Read the model definition and answer for the solid it produces. Units are mm, in the model's axes. A direction names the side the tool comes from. Round coordinates to 2 decimals unless told otherwise and drop trailing zeros. Order: outer loops, then holes, each group sorted by start corner. A loop starts at its lowest first (then second) coordinate and runs counter-clockwise, first axis right, second up.
Autodesk Inventor part; units mm, degrees
ref_plane "YZ Plane" through (0, 0, 0) normal (1, 0, 0) x (0, 1, 0)
ref_plane "XZ Plane" through (0, 0, 0) normal (0, 1, 0) x (-1, 0, 0)
ref_plane "XY Plane" through (0, 0, 0) normal (0, 0, 1) x (1, 0, 0)
sketch "Sketch1" plane through (0, 0, 0) normal (0, 1, 0) x (-1, 0, 0)
  line L0 (-166.6875, 104.5) -> (166.6875, 104.5)
  line L1 (166.6875, -104.5) -> (-166.6875, -104.5)
  line L2 (-166.6875, 104.5) -> (166.6875, -104.5) construction
  line L3 (166.6875, 104.5) -> (-166.6875, -104.5) construction
  line L4 (166.6875, 88.5) -> (-166.6875, 88.5)
  line L5 (166.6875, -88.5) -> (-166.6875, -88.5)
  line L6 (120.9675, 104.5) -> (120.9675, -104.5)
  line L7 (-120.9675, 104.5) -> (-120.9675, -104.5)
  line L8 (-109.9675, 104.5) -> (-109.9675, -104.5)
  line L9 (-131.9675, 104.5) -> (-131.9675, -104.5)
  circle A0 centre (-109.9675, 88.5) radius 1.85
  circle A1 centre (-131.9675, 88.5) radius 1.85
  circle A2 centre (-109.9675, -88.5) radius 1.85
  circle A3 centre (-131.9675, -88.5) radius 1.85
  line L10 (131.9675, 104.5) -> (131.9675, -104.5)
  line L11 (109.9675, 104.5) -> (109.9675, -104.5)
  circle A4 centre (131.9675, 88.5) radius 1.85
  circle A5 centre (131.9675, -88.5) radius 1.85
  line L12 (-109.9675, 104.5) -> (-109.9675, -104.5)
  circle A6 centre (109.9675, 88.5) radius 1.85
  circle A7 centre (109.9675, -88.5) radius 1.85
  line L13 (-104.9675, 71.5) -> (-1.9675, 71.5)
  line L14 (-1.9675, 71.5) -> (-1.9675, -71.5)
  line L15 (-1.9675, -71.5) -> (-104.9675, -71.5)
  line L16 (-104.9675, -71.5) -> (-104.9675, 71.5)
  line L17 (175.9652, 0) -> (-157.4098, 0)
  line L18 (104.9675, 71.5) -> (1.9675, 71.5)
  line L19 (1.9675, 71.5) -> (1.9675, -71.5)
  line L20 (1.9675, -71.5) -> (104.9675, -71.5)
  line L21 (104.9675, -71.5) -> (104.9675, 71.5)
  line L22 (9.4675, 64) -> (97.4675, 64)
  line L23 (97.4675, 64) -> (97.4675, -64)
  line L24 (97.4675, -64) -> (9.4675, -64)
  line L25 (9.4675, -64) -> (9.4675, 64)
  line L26 (-9.4675, 64) -> (-97.4675, 64)
  line L27 (-97.4675, 64) -> (-97.4675, -64)
  line L28 (-97.4675, -64) -> (-9.4675, -64)
  line L29 (-9.4675, -64) -> (-9.4675, 64)
  circle A8 centre (-9.4675, 64) radius 1.85
  circle A9 centre (-9.4675, -64) radius 1.85
  circle A10 centre (-97.4675, 64) radius 1.85
  circle A11 centre (-97.4675, -64) radius 1.85
  circle A12 centre (97.4675, 64) radius 1.85
  circle A13 centre (97.4675, -64) radius 1.85
  circle A14 centre (9.4675, -64) radius 1.85
  circle A15 centre (9.4675, 64) radius 1.85
  line L30 (-158.6875, 71.5) -> (-144.9675, 71.5)
  line L31 (-136.9675, 63.5) -> (-136.9675, -63.5)
  line L32 (-144.9675, -71.5) -> (-158.6875, -71.5)
  arc A16 (-136.9675, 63.5) -> (-144.9675, 71.5) centre (-144.9675, 63.5) ccw
  arc A17 (-144.9675, -71.5) -> (-136.9675, -63.5) centre (-144.9675, -63.5) ccw
  line L33 (-166.6875, -104.5) -> (-166.6875, -79.5)
  line L34 (-166.6875, 79.5) -> (-166.6875, 104.5)
  arc A18 (-166.6875, 79.5) -> (-158.6875, 71.5) centre (-158.6875, 79.5) ccw
  arc A19 (-158.6875, -71.5) -> (-166.6875, -79.5) centre (-158.6875, -79.5) ccw
  line L35 (158.6875, 71.5) -> (144.9675, 71.5)
  line L36 (136.9675, 63.5) -> (136.9675, -63.5)
  line L37 (144.9675, -71.5) -> (158.6875, -71.5)
  arc A20 (144.9675, 71.5) -> (136.9675, 63.5) centre (144.9675, 63.5) ccw
  arc A21 (136.9675, -63.5) -> (144.9675, -71.5) centre (144.9675, -63.5) ccw
  line L38 (166.6875, 104.5) -> (166.6875, 79.5)
  line L39 (166.6875, -79.5) -> (166.6875, -104.5)
  arc A22 (158.6875, 71.5) -> (166.6875, 79.5) centre (158.6875, 79.5) ccw
  arc A23 (166.6875, -79.5) -> (158.6875, -71.5) centre (158.6875, -79.5) ccw
  point P0 (0, 0)
  dimension "d0" = 209
  dimension "d6" = 22
  dimension "d8" = 3.7
  dimension "d11" = 22
  dimension "d19" = 16
  dimension "d20" = 16
  dimension "d24" = 143
  dimension "d25" = 103
  dimension "d26" = 16
  dimension "d27" = 143
  dimension "d28" = 103
  dimension "d29" = 16
  dimension "d30" = 7.5
  dimension "d31" = 7.5
  dimension "d34" = 3.7
  dimension "d36" = 8
  dimension "d39" = 16
  dimension "d40" = 143
  dimension "d41" = 333.375
  dimension "d42" = 45.72
  dimension "d45" = 45.72
  dimension "d48" = 16
  dimension "d49" = 143
  dimension "d50" = 553.31
  dimension "d51" = 9.2777
extrude "Extrusion1" add sketch "Sketch1" along normal blind 6.35 contours L0 L9 A1 L4 L34 | L0 L7 L4 A1 L9 | L4 A1 L9 L17 L31 A16 L30 A18 L34 | L0 L8 A0 L4 L7 | L0 L11 A6 L4 A0 L8 | L7 L17 L9 A1 L4 | L4 A0 L8 L17 L7 | L0 L6 L4 A6 L11 | L17 L8 A2 L5 L7 | L7 L5 A3 L9 L17 | L9 A3 L5 L33 A19 L32 A17 L31 L17 | L0 L10 A4 L4 L6 | L4 A6 L11 L17 L21 L18 L19 L14 L13 L16 L8 A0 | L7 L1 L9 A3 L5 | L5 A2 L8 L1 L7 | L17 L16 L15 L14 L19 L20 L21 L11 A7 L5 A2 L8 | L0 L38 L4 A4 L10 | L6 L17 L11 A6 L4 | L4 A4 L10 L17 L6 | L17 L27 A11 L28 A9 L29 L14 L15 L16 | L16 L13 L14 L17 L29 A8 L26 A10 L27 | A3 L9 L1 L33 L5 | L17 L10 A5 L5 L6 | L6 L5 A7 L11 L17 | A2 L5 A7 L11 L1 L8 | L27 A10 L26 A8 L29 L17 | L17 L29 A9 L28 A11 L27 | L38 A22 L35 A20 L36 L17 L10 A4 L4 | L6 L1 L11 A7 L5 | L5 A5 L10 L1 L6 | L17 L36 A21 L37 A23 L39 L5 A5 L10 | L21 L20 L19 L17 L25 A14 L24 A13 L23 | L17 L23 A12 L22 A15 L25 L19 L18 L21 | A5 L5 L39 L1 L10 | L23 A13 L24 A14 L25 L17 | L17 L25 A15 L22 A12 L23
properties part number "BasePlate"
Q1. A cutting plane is placed at B-B, the plane z = 14. Give the vertices of the cut face in (x, y), plus the area to 3 significant figures.
Outcome:
outline: (-136.97, 0) - (136.97, 0) - (136.97, 6.35) - (-136.97, 6.35) - close
area: 1,740 mm2
Q2. A cutting plane is placed at A-A, the plane y = 1.25. Give the number of separate pieces and of enclosed holes in the cut face, plus the area to 3 significant figures.
Outcome:
separate pieces: 1
enclosed holes: 16
area: 61,000 mm2
Q3. For a pull along Z with two mould halves and no side action, classify faces 4 (the face through (2, 3, 104.5)), 5 (the face through (164.3, 3.1, 73.8)), 6 (the face through (2, 0, 1)) as released by +Z, released by -Z, zero draft, split by the parting line, or undercut.
Outcome:
face 4: released by +Z
face 5: undercut
face 6: zero draft
Q4. A flat-ended cylindrical pin translates along its axis: pin 1 (2 mm diameter, centred on x = -131.97, z = 88.5, fed in from -Y). Find the tip coordinate at first contact, or state that the pin passes through.
Outcome:
pin 1: passes through
Q5. Straight lines are drawn through the part: probe 1 along X at (y, z) = (2.75, 88.5); probe 2 along Z at (x, y) = (98, 0.75); probe 3 along X at (y, z) = (2.5, -64). For each, find the intervals that lie inside material, in ascending order.
Outcome:
probe 1: x = -166.69 to -133.82, -130.12 to -111.82, -108.12 to 108.12, 111.82 to 130.12, 133.82 to 166.69
probe 2: z = -104.5 to -65.77, -62.23 to 62.23, 65.77 to 104.5
probe 3: x = -136.98 to -99.32, -95.62 to -11.32, -7.62 to 7.62, 11.32 to 95.62, 99.32 to 136.98
Q6. For faces 1 (the face through (2, 6.35, 1)), 2 (the face through (139.249, 3.131, -69.094)), 3 (the face through (-164.4, 3.1, 73.9)), determine the directions among +Z, -Z, +X, -X, +Y, -Y from which every point of the face is accessible in a straight line to the end or side of a thin tool.
Outcome:
face 1: +Z, -Z, +X, -X, +Y
face 2: +X, +Y, -Y
face 3: -X, +Y, -Y
